Part model, mm, in its own coordinate system. Round coordinates to 2 decimals unless told otherwise and drop trailing zeros. Write each loop counter-clockwise with the first axis right and the second up, starting at its lowest first coordinate (ties: lowest second). Pieces come first, ordered by that corner, then holes.
```python
from build123d import *

# Parameters (mm, degrees)
SKETCH2_R           = 4.7625
SKETCH2_R_2         = 12.8
BOSS_EXTRUDE2_DEPTH = 5.334
SKETCH3_R           = 6.35
SKETCH3_R_2         = 4.7625
CUT_EXTRUDE3_DEPTH  = 2.667
SKETCH3_2_R         = 4.7625
CUT_EXTRUDE4_DEPTH  = 6.334


with BuildPart() as part:
    # Sketch2 → Boss-Extrude2 (new body)
    with BuildSketch(Plane.XY):
        Polygon((-55.022779977, 2.330692017), (-24, -20.208676973), (24, -20.208676973), (55.022779977, 2.330692017), (34.005948181, 67.013849238), (-34.005948181, 67.013849238), align=None)
        Circle(SKETCH2_R, mode=Mode.SUBTRACT)
        with Locations((-24, 20.208676973)):
            Circle(SKETCH2_R_2, mode=Mode.SUBTRACT)
        with Locations((24, 20.208676973)):
            Circle(SKETCH2_R_2, mode=Mode.SUBTRACT)
    extrude(amount=BOSS_EXTRUDE2_DEPTH)

    # Sketch3 → Cut-Extrude3 (cut)
    with BuildSketch(Plane.XY.offset(5.334)):
        Circle(SKETCH3_R)
        Circle(SKETCH3_R_2, mode=Mode.SUBTRACT)
        with Locations((45.751679669, 9.848845061)):
            Circle(SKETCH3_R)
        with Locations((45.751679669, 9.848845061)):
            Circle(SKETCH3_R_2, mode=Mode.SUBTRACT)
        with Locations((0, 33.008676973)):
            Circle(SKETCH3_R)
        with Locations((0, 33.008676973)):
            Circle(SKETCH3_R_2, mode=Mode.SUBTRACT)
        with Locations((-45.751679669, 9.848845061)):
            Circle(SKETCH3_R)
        with Locations((-45.751679669, 9.848845061)):
            Circle(SKETCH3_R_2, mode=Mode.SUBTRACT)
    extrude(amount=-CUT_EXTRUDE3_DEPTH, mode=Mode.SUBTRACT)

    # Sketch3_2 → Cut-Extrude4 (cut, through all)
    with BuildSketch(Plane.XY.offset(5.334)):
        with Locations((-45.751679669, 9.848845061)):
            Circle(SKETCH3_2_R)
        with Locations((0, 33.008676973)):
            Circle(SKETCH3_2_R)
        with Locations((45.751679669, 9.848845061)):
            Circle(SKETCH3_2_R)
    extrude(amount=-CUT_EXTRUDE4_DEPTH, mode=Mode.SUBTRACT)


solid = part.part
```
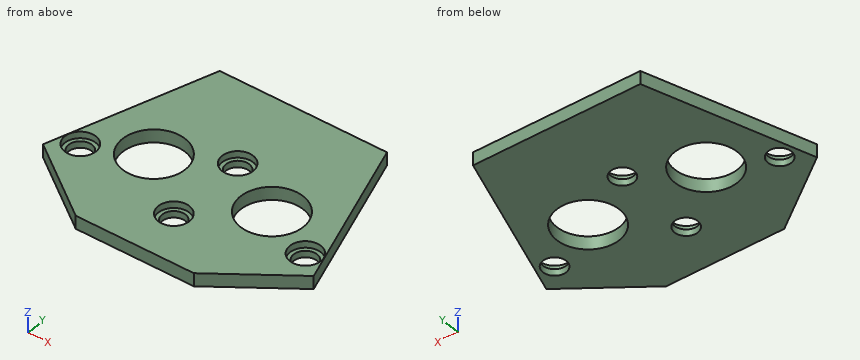
Q1. Cut at B-B on y = 31.5. Write the cut outline in (x, z).
Values follow:
outline: (-45.55, 0) - (-30.03, 0) - (-30.03, 5.33) - (-45.55, 5.33) - close; (-17.97, 0) - (-4.52, 0) - (-4.52, 2.67) - (-6.17, 2.67) - (-6.17, 5.33) - (-17.97, 5.33) - close; (4.52, 0) - (17.97, 0) - (17.97, 5.33) - (6.17, 5.33) - (6.17, 2.67) - (4.52, 2.67) - close; (30.03, 0) - (45.55, 0) - (45.55, 5.33) - (30.03, 5.33) - close
Q2. Drop flat-ended pins along their axis: pin 1 (15.5 mm diameter, centred on x = 24, y = 20.21, fed in from +Z); pin 2 (1.5 mm diameter, centred on y = 23.5, z = 3.5, fed in from -X); pin 3 (11.5 mm diameter, centred on x = 0, y = 33.01, fed in from +Z); pin 4 (2 mm diameter, centred on y = -9, z = 5, fed in from +X). Give the stop position or say it passes through.
Values follow:
pin 1: passes through
pin 2: stops at x = -48.39
pin 3: stops at z = 2.67
pin 4: stops at x = 40.8
Q3. Wall check: L1, parallel to Y at x = 0, z = 4.75; L2, parallel to Y at x = 24, z = 4.1; L3, parallel to X at y = 10, z = 0.8. Give the ranges that are in metal, low to high.
Values follow:
L1: y = -20.21 to -6.35, 6.35 to 26.66, 39.36 to 67.01
L2: y = -20.21 to 7.41, 33.01 to 67.01
L3: x = -52.53 to -50.51, -40.99 to -31.72, -16.28 to 16.28, 31.72 to 40.99, 50.51 to 52.53
Q4. Cut at A-A on x = 0. Write the cut outline in (y, z), plus the area to 3 significant figures.
Values follow:
outline: (-20.21, 0) - (-4.76, 0) - (-4.76, 2.67) - (-6.35, 2.67) - (-6.35, 5.33) - (-20.21, 5.33) - close; (4.76, 0) - (28.25, 0) - (28.25, 2.67) - (26.66, 2.67) - (26.66, 5.33) - (6.35, 5.33) - (6.35, 2.67) - (4.76, 2.67) - close; (37.77, 0) - (67.01, 0) - (67.01, 5.33) - (39.36, 5.33) - (39.36, 2.67) - (37.77, 2.67) - close
area: 347 mm2
Q5. Cut at C-C on y = 0. Write the cut outline in (x, z).
Values follow:
outline: (-51.81, 0) - (-4.76, 0) - (-4.76, 2.67) - (-6.35, 2.67) - (-6.35, 5.33) - (-51.81, 5.33) - close; (4.76, 0) - (51.81, 0) - (51.81, 5.33) - (6.35, 5.33) - (6.35, 2.67) - (4.76, 2.67) - close
Q6. Cut at D-D on z = 1. Write the cut outline in (x, y) (1 decimal), plus the area to 3 significant figures.
Values follow:
outline: (-55, 2.3) - (-24, -20.2) - (24, -20.2) - (55, 2.3) - (34, 67) - (-34, 67) - close; hole circle Ø9.5 at (-45.8, 9.8); hole circle Ø25.6 at (-24, 20.2); hole circle Ø9.5 at (0, 0); hole circle Ø9.5 at (0, 33); hole circle Ø25.6 at (24, 20.2); hole circle Ø9.5 at (45.8, 9.8)
area: 6,230 mm2
